from build123d import *

# Parameters (mm, degrees)
SKETCH_1_R      = 2.05
SKETCH_1_R_2    = 3.55
SKETCH_1_R_3    = 9.55
SKETCH_1_W      = 8.1
SKETCH_1_H      = 2.1
EXTRUDE_1_DEPTH = 2


with BuildPart() as part:
    # 草图1 → 凸台-拉伸1 (new body)
    with BuildSketch(Plane.XY):
        Polygon((81, -15.149736791), (81, 7.149736791), (40.992999038, 17.149736791), (12.70872779, 17.149736791), (-19, 7.149736791), (-19, -15.149736791), (12.70872779, -25.149736791), (40.992999038, -25.149736791), align=None)
        Circle(SKETCH_1_R, mode=Mode.SUBTRACT)
        with Locations((62, 0)):
            Circle(SKETCH_1_R, mode=Mode.SUBTRACT)
        with Locations((62, -8)):
            Circle(SKETCH_1_R, mode=Mode.SUBTRACT)
        with Locations((0, -8)):
            Circle(SKETCH_1_R, mode=Mode.SUBTRACT)
        with Locations((45.142135624, 10.142135624)):
            Circle(SKETCH_1_R, mode=Mode.SUBTRACT)
        with Locations((45.142135624, -18.142135624)):
            Circle(SKETCH_1_R, mode=Mode.SUBTRACT)
        with Locations((16.857864376, -18.142135624)):
            Circle(SKETCH_1_R, mode=Mode.SUBTRACT)
        with Locations((16.857864376, 10.142135624)):
            Circle(SKETCH_1_R, mode=Mode.SUBTRACT)
        with Locations((74, 0)):
            Circle(SKETCH_1_R_2, mode=Mode.SUBTRACT)
        with Locations((74, -8)):
            Circle(SKETCH_1_R_2, mode=Mode.SUBTRACT)
        with Locations((-12, -8)):
            Circle(SKETCH_1_R_2, mode=Mode.SUBTRACT)
        with Locations((-12, 0)):
            Circle(SKETCH_1_R_2, mode=Mode.SUBTRACT)
        with Locations((31, -4)):
            Circle(SKETCH_1_R_3, mode=Mode.SUBTRACT)
        with Locations((15, 0)):
            Rectangle(SKETCH_1_W, SKETCH_1_H, mode=Mode.SUBTRACT)
        with Locations((47, 0)):
            Rectangle(SKETCH_1_W, SKETCH_1_H, mode=Mode.SUBTRACT)
        with Locations((47, -8)):
            Rectangle(SKETCH_1_W, SKETCH_1_H, mode=Mode.SUBTRACT)
        with Locations((15, -8)):
            Rectangle(SKETCH_1_W, SKETCH_1_H, mode=Mode.SUBTRACT)
    extrude(amount=EXTRUDE_1_DEPTH)


solid = part.part
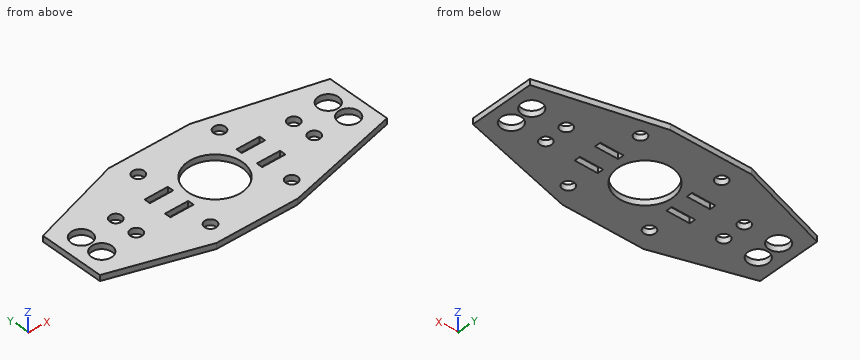
Source: CAD feature listing. Evaluate the final solid. Frame: model axes, mm. Round coordinates to 2 decimals unless told otherwise and drop trailing zeros. Order: outer loops, then holes, each group sorted by start corner. A loop starts at its lowest first (then second) coordinate and runs counter-clockwise, first axis right, second up. Notation, with made-up numbers: (44.5, -29.75) -> (52.5, -29.75) arc R19 ccw to (52.5, -8.75) -> close; hole circle Ø8 at (1.5, 30). An arc over 180 degrees is marked (long way). Answer as CSV lines item,"result".
Item 1: Pin query (flat end, axial travel): pin 1 Ø2.5 at (x, y) = (0, 0) entering from +Z; pin 2 Ø0.6 at (x, z) = (48, 1.5) entering from +Y. Return the tip coordinate at first contact, or that it passes through.
A:
pin 1,"through"
pin 2,"y = 15.47"
Item 2: Section B-B, the plane x = 16.5. Return loops of the section in (y, z).
A:
outline,"(-25.15, 0) -> (-20.16, 0) -> (-20.16, 2) -> (-25.15, 2) -> close; (-16.12, 0) -> (-9.05, 0) -> (-9.05, 2) -> (-16.12, 2) -> close; (-6.95, 0) -> (-1.05, 0) -> (-1.05, 2) -> (-6.95, 2) -> close; (1.05, 0) -> (8.12, 0) -> (8.12, 2) -> (1.05, 2) -> close; (12.16, 0) -> (17.15, 0) -> (17.15, 2) -> (12.16, 2) -> close"
Item 3: Section C-C, the plane y = -8. Count the separate pieces of the cut face and the enclosed holes in it, plus the area to 3 significant figures.
A:
separate pieces,"8"
enclosed holes,"0"
area,"88.1 mm²"
Item 4: Section A-A, the plane x = 73.5. Return loops of the section in (y, z), plus the area to 3 significant figures.
A:
outline,"(-17.02, 0) -> (-11.51, 0) -> (-11.51, 2) -> (-17.02, 2) -> close; (-4.49, 0) -> (-3.51, 0) -> (-3.51, 2) -> (-4.49, 2) -> close; (3.51, 0) -> (9.02, 0) -> (9.02, 2) -> (3.51, 2) -> close"
area,"24.0 mm²"
Item 5: Line query: L1, parallel to Y at x = 71, z = 0.6; L2, parallel to Y at x = 74, z = 0.7; L3, parallel to Y at x = 31, z = 1.4. Output: solid intervals per line, ascending.
A:
L1,"-17.65 to -9.9, -6.1 to -1.9, 1.9 to 9.65"
L2,"-16.9 to -11.55, -4.45 to -3.55, 3.55 to 8.9"
L3,"-25.15 to -13.55, 5.55 to 17.15"
